CAD build for the part. Positions are in the model's coordinates, mm. A direction names the side the tool comes from. Coordinates: 2 decimals unless noted, no trailing zeros. Order: outer loops, then holes, each group sorted by start corner. A loop starts at its lowest first (then second) coordinate and runs counter-clockwise, first axis right, second up. Notation, with made-up numbers: (14.5, 21.25) -> (29.5, 21.25) arc R11 ccw to (29.5, 25.25) -> close; hole circle Ø6 at (-3.75, 55). An arc over 180 degrees is marked (long way). Use one line per item in the form item = value. Start each with the question number.
Autodesk Inventor part; units mm, degrees
ref_plane "YZ Plane" through (0, 0, 0) normal (1, 0, 0) x (0, 1, 0)
ref_plane "XZ Plane" through (0, 0, 0) normal (0, 1, 0) x (-1, 0, 0)
ref_plane "XY Plane" through (0, 0, 0) normal (0, 0, 1) x (1, 0, 0)
sketch "Sketch1" plane through (0, 0, 0) normal (0, 1, 0) x (-1, 0, 0)
  line L0 (0, 0) -> (304.8, 0)
  line L1 (304.8, 0) -> (304.8, 254)
  line L2 (304.8, 254) -> (0, 254)
  line L3 (0, 254) -> (0, 0)
  line L4 (301.625, 250.825) -> (301.625, 3.175)
  line L5 (301.625, 3.175) -> (3.175, 3.175)
  line L6 (3.175, 3.175) -> (3.175, 250.825)
  line L7 (3.175, 250.825) -> (301.625, 250.825)
  dimension "d0" = 304.8
  dimension "d1" = 254
  dimension "d21" = 3.175
extrude "Extrusion1" add sketch "Sketch1" along normal blind 92.71
sketch "Sketch5" plane through (0, 0, 0) normal (0, -1, 0) x (1, 0, 0)
  line L0 (0, 0) -> (-304.8, 0)
  line L1 (-304.8, 0) -> (-304.8, 254)
  line L2 (-304.8, 254) -> (0, 254)
  line L3 (0, 254) -> (0, 0)
  dimension "d22" = 304.8
  dimension "d23" = 254
extrude "Extrusion4" add sketch "Sketch5" along normal blind 3.175
properties part number "Lower Chassis"
1) Cut at C-C on x = -251.5. Give the cut face in (y, z) (3 decimals), then the cut area to 3 significant figures.
2) 3-axis set-ups, long thin cutter, end or side, ignore diameter. For faces 5 (the face through (-150, 44, 0)), 6 (the face through (-301.625, 46, 129)): which of +Z, -Z, +X, -X, +Y, -Y reach the whole face in a straight line?
3) Cut at A-A on z = 30. Give the cut face in (x, y) (3 decimals), then the cut area to 3 significant figures.
4) Cut at B-B on y = 51.5. Give the cut face in (x, z) (3 decimals).
5) Drop flat-ended pins along their axis: P1, Ø12, axis at x = -71.5, z = 120, coming from the +Y side; P2, Ø1, axis at x = -254.5, y = 7, coming from the -Z side. Give the stop position or say it passes through.
6) Probe L1, parallel to X at y = 58.5, z = 212.5 (3 decimals); L2, parallel to Z at x = -248, y = 64 (3 decimals); L3, parallel to Y at x = -251.5, z = 125 (3 decimals). List the from-to ranges inside material, lowest first.
7) Two-plate mould, pull along Z, no slides. Class faces 1 (the face through (-3.175, 46, 125)), 2 (the face through (-154, 46, 3.175)), 3 (the face through (-155, 44, 254)), 4 (the face through (-304.8, 44, 125)): released by +Z, released by -Z, zero draft, split by the parting line, or undercut.
Values follow:
q1.outline = (-3.175, 0) -> (92.71, 0) -> (92.71, 3.175) -> (0, 3.175) -> (0, 250.825) -> (92.71, 250.825) -> (92.71, 254) -> (-3.175, 254) -> close
q1.area = 1,400 mm^2
q2.face_5 = -Z, +X, -X, +Y, -Y
q2.face_6 = +Y
q3.outline = (-304.8, -3.175) -> (0, -3.175) -> (0, 92.71) -> (-3.175, 92.71) -> (-3.175, 0) -> (-301.625, 0) -> (-301.625, 92.71) -> (-304.8, 92.71) -> close
q3.area = 1,560 mm^2
q4.outline = (-304.8, 0) -> (0, 0) -> (0, 254) -> (-304.8, 254) -> close; hole (-301.625, 3.175) -> (-3.175, 3.175) -> (-3.175, 250.825) -> (-301.625, 250.825) -> close
q5.P1 = 0
q5.P2 = 0
q6.L1 = -304.8 to -301.625, -3.175 to 0
q6.L2 = 0 to 3.175, 250.825 to 254
q6.L3 = -3.175 to 0
q7.face_1 = undercut
q7.face_2 = undercut
q7.face_3 = released by +Z
q7.face_4 = zero draft
